```python
from build123d import *

# Parameters (mm, degrees)
SKETCH1_W           = 60
SKETCH1_H           = 30
BOSS_EXTRUDE1_DEPTH = 150
SKETCH2_R           = 25
CUT_EXTRUDE1_DEPTH  = 30
FILLET1_R           = 30


with BuildPart() as part:
    # Sketch1 → Boss-Extrude1 (new body)
    with BuildSketch(Plane(origin=(0, 0, 0), x_dir=(0, 0, -1), z_dir=(1, 0, 0))):
        Rectangle(SKETCH1_W, SKETCH1_H)
    extrude(amount=BOSS_EXTRUDE1_DEPTH)

    # Sketch2 → Cut-Extrude1 (cut)
    with BuildSketch(Plane(origin=(0, 15, 0), x_dir=(1, 0, 0), z_dir=(0, 1, 0))):
        with Locations(Location((120, 0, 0), (0, 0, 270))):
            Circle(SKETCH2_R)
    extrude(amount=-CUT_EXTRUDE1_DEPTH, mode=Mode.SUBTRACT)

    # Fillet1
    fillet1_edges = [part.edges().sort_by_distance(p)[0] for p in [
        (150, 0, -30),
        (150, 0, 30),
    ]]
    fillet(fillet1_edges, radius=FILLET1_R - 0.0001)  # a hair under: the kernel refuses the full size


solid = part.part
```
Geometry check sheet. Reference: the model listing, model coordinates, mm. Coordinates: 2 decimals unless noted, no trailing zeros. Order: outer loops, then holes, each group sorted by start corner. A loop starts at its lowest first (then second) coordinate and runs counter-clockwise, first axis right, second up.
Item 1: Mould release check, pull along Z, two halves, no side actions. Record for faces 1 (the cylindrical face through (140.979, 0.21, 21.445)), 2 (the cylindrical face through (144.787, 0.21, -3.255)), 3 (the flat face through (59, 0, -30)), 4 (the flat face through (57, -15, 0)): released by +Z, released by -Z, zero draft, split by the parting line, or undercut.
Item 2: Depth check by flat-ended pin: pin 1 (1.5 mm diameter, centred on y = -5.5, z = 16.5, fed in from +X); pin 2 (1.5 mm diameter, centred on y = -10.5, z = 20, fed in from +X); pin 3 (2 mm diameter, centred on y = 6, z = -4, fed in from +X). Enter the tip coordinate at first touch or a pass-through.
Item 3: Section check C-C (z = -7.5). Enter the section's corners in (x, y), plus the area to 3 significant figures.
Item 4: Scan lines: line 1 along X through (y, z) = (-4.25, 0); line 2 along X through (y, z) = (8.5, -5); line 3 along Z through (x, y) = (98.5, 9.75). Record each from-to range of solid material in increasing order.
Item 5: Section check B-B (z = -22.5). Enter the section's corners in (x, y).
Check sheet entries:
1. face 1: released by +Z
1. face 2: undercut
1. face 3: released by -Z
1. face 4: zero draft
2. pin 1: stops at x = 145.53
2. pin 2: stops at x = 143.01
2. pin 3: stops at x = 149.85
3. outline: (0, -15) - (96.15, -15) - (96.15, 15) - (0, 15) - close; (143.85, -15) - (149.05, -15) - (149.05, 15) - (143.85, 15) - close
3. area: 3,040 mm2
4. line 1: x = 0 to 95, 145 to 150
4. line 2: x = 0 to 95.51, 144.49 to 149.58
4. line 3: z = -30 to -12.76, 12.76 to 30
5. outline: (0, -15) - (109.1, -15) - (109.1, 15) - (0, 15) - close; (130.9, -15) - (139.84, -15) - (139.84, 15) - (130.9, 15) - close
